from build123d import *

# Parameters (mm, degrees)
F0_W     = 30
F0_H     = 30
F1_DEPTH = 60
F2_R     = 8
F3_DEPTH = 30.001
F3_TAPER = -3
F4_R     = 6
F5_DEPTH = 9


with BuildPart() as f1:
    # F0 (on Front) → F1 (new body)
    with BuildSketch(Plane.XZ):
        Rectangle(F0_W, F0_H)
    extrude(amount=F1_DEPTH)

    # F2 (on face) → F3 (cut, through all)
    with BuildSketch(Plane.YZ.offset(15)):
        with Locations((-20, 0)):
            Circle(F2_R)
    extrude(amount=-F3_DEPTH, taper=F3_TAPER, mode=Mode.SUBTRACT)

    # F4 (on face) → F5 (cut)
    with BuildSketch(Plane.XZ.offset(60)):
        Circle(F4_R)
    extrude(amount=-F5_DEPTH, mode=Mode.SUBTRACT)


solid = f1.part
Input: part model. Units: mm. Frame: model coordinates. A direction names the side the tool comes from. Round coordinates to 2 decimals unless told otherwise and drop trailing zeros. Write each loop counter-clockwise with the first axis right and the second up, starting at its lowest first coordinate (ties: lowest second). Pieces come first, ordered by that corner, then holes.
1) Reachability of faces 4 (the cylindrical face through (-6, -56, 0)), 5 (the conical face through (-0.21, -28.79, 0.39)) from +Z, -Z, +X, -X, +Y, -Y: full face, straight path, thin tool, end or side. Return the list, or none.
2) Cut plane B-B (y = -56). Return the cut outline in (x, z).
3) Cut plane D-D (x = -11). Return the cut outline in (y, z).
4) Cut plane C-C (x = 2). Return the cut outline in (y, z), then the cut area to 3 significant figures.
5) Contact query for a flat-ended pin moving along its axis: P1, Ø6, axis at x = -2, z = -2, coming from the -Y side. Output: stop coordinate, or through.
6) Cut plane A-A (y = -20). Return the cut outline in (x, z).
7) Ray query, L1, parallel to Z at x = 0, y = -56; L2, parallel to Z at x = -5.5, y = -18.5; L3, parallel to Y at x = 13, z = -2. Return the intervals inside material, ascending.
8) Draft query along Z for faces 1 (the flat face through (0, -51, 0)), 2 (the flat face through (0, -30, -15)), 3 (the flat face through (-15, -30, 0)). Return one class per face: pulls with the +Z half, pulls with the -Z half, needs draft (parallel to the pull), parting line crosses it, or undercut.
Geometry says:
1. face 4: -Y
1. face 5: -X
2. outline: (-15, -15) - (15, -15) - (15, 15) - (-15, 15) - close; hole circle Ø12 at (0, 0)
3. outline: (-60, -15) - (0, -15) - (0, 15) - (-60, 15) - close; hole circle Ø18.73 at (-20, 0)
4. outline: (-60, -15) - (0, -15) - (0, 15) - (-60, 15) - (-60, 5.66) - (-51, 5.66) - (-51, -5.66) - (-60, -5.66) - close; hole circle Ø17.36 at (-20, 0)
4. area: 1,460 mm2
5. P1: stops at y = -51
6. outline: (-15, -15) - (15, -15) - (15, -8) - (-15, -9.57) - close; (-15, 9.57) - (15, 8) - (15, 15) - (-15, 15) - close
7. L1: z = -15 to -6, 6 to 15
7. L2: z = -15 to -8.95, 8.95 to 15
7. L3: y = -60 to -27.85, -12.15 to 0
8. face 1: undercut
8. face 2: pulls with the -Z half
8. face 3: needs draft
